Here's how the part is built. I have some questions about the finished solid (model axes, mm). Round coordinates to 2 decimals unless told otherwise and drop trailing zeros. Order: outer loops, then holes, each group sorted by start corner. A loop starts at its lowest first (then second) coordinate and runs counter-clockwise, first axis right, second up. Notation, with made-up numbers: M -19,-34.75 L 19,-34.75 A4 ccw 19,-27.75 Z; hole C 73.25,10.5 d1. An arc over 180 degrees is marked long. Answer as CSV lines item,"result". Start each with the question number.
```python
from build123d import *

# Parameters (mm, degrees)
SKETCH1_W          = 76.2
SKETCH1_H          = 44.45
BASE_FLANGE1_DEPTH = 4.55422
CUT_EXTRUDE1_DEPTH = 45.342998825
FILLET1_R          = 4.7625
FILLET2_R          = 12.7
SKETCH3_R          = 3.175
CUT_EXTRUDE2_DEPTH = 45.342998825
FILLET3_R          = 6.35
CUT_EXTRUDE3_DEPTH = 45.342998825


# Sheet-metal steps are written as plain solids
with BuildPart() as part:
    # Sketch1 → Base-Flange1 (new body)
    with BuildSketch(Plane.XY):
        Rectangle(SKETCH1_W, SKETCH1_H)
    extrude(amount=BASE_FLANGE1_DEPTH)

    # Sketch2 → Cut-Extrude1 (cut, through all)
    with BuildSketch(Plane.XY.offset(4.55422)):
        Polygon((12.7, 22.225), (38.1, 15.419090512), (38.1, 22.225), align=None)
    extrude(amount=-CUT_EXTRUDE1_DEPTH, mode=Mode.SUBTRACT)

    # Fillet1
    fillet1_edges = [part.edges().sort_by_distance(p)[0] for p in [
        (-38.1, 22.225, 2.27711),
    ]]
    fillet(fillet1_edges, radius=FILLET1_R)

    # Fillet2
    fillet2_edges = [part.edges().sort_by_distance(p)[0] for p in [
        (12.7, 22.225, 2.27711),
        (38.1, 15.419090512, 2.27711),
    ]]
    fillet(fillet2_edges, radius=FILLET2_R)

    # Sketch3 → Cut-Extrude2 (cut, through all)
    with BuildSketch(Plane.XY.offset(4.55422)):
        with Locations((0, -9.525)):
            Circle(SKETCH3_R)
        with Locations((25.4, -9.525)):
            Circle(SKETCH3_R)
    extrude(amount=-CUT_EXTRUDE2_DEPTH, mode=Mode.SUBTRACT)

    # Fillet3
    fillet3_edges = [part.edges().sort_by_distance(p)[0] for p in [
        (38.1, -22.225, 2.27711),
        (-38.1, -22.225, 2.27711),
    ]]
    fillet(fillet3_edges, radius=FILLET3_R)

    # Sketch4 → Cut-Extrude3 (cut, through all)
    with BuildSketch(Plane.XY.offset(4.55422)):
        with BuildLine():
            Line((-3.175, -9.525), (-3.175, -3.175))
            ThreePointArc((-3.175, -3.175), (0, 0), (3.175, -3.175))
            Line((3.175, -3.175), (3.175, -9.525))
            ThreePointArc((3.175, -9.525), (0, -12.7), (-3.175, -9.525))
        make_face()
        with BuildLine():
            Line((22.225, -9.525), (22.225, -3.175))
            ThreePointArc((22.225, -3.175), (25.4, 0), (28.575, -3.175))
            Line((28.575, -3.175), (28.575, -9.525))
            ThreePointArc((28.575, -9.525), (25.4, -12.7), (22.225, -9.525))
        make_face()
    extrude(amount=-CUT_EXTRUDE3_DEPTH, mode=Mode.SUBTRACT)


solid = part.part
```
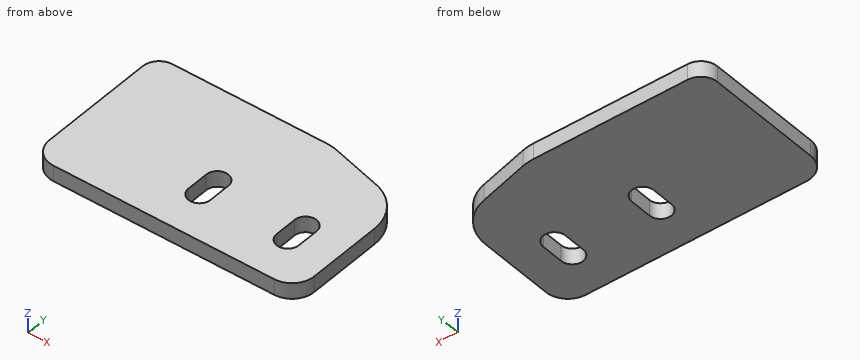
Item 1: If we section it at C-C on x = 25.4: Please give me the cut outline in (y, z) (3 decimals).
Item 2: If we section it at D-D on y = 11.5: Please give me the cut outline in (x, z), and give its area (3 significant figures).
Item 3: For P1, Ø1.5, axis at x = 22, z = 3, coming from the +Y side, with a flat end and sliding along its axis, tell me the tip position at first contact or that it passes through.
Item 4: If we section it at B-B on z = 1.45: Count the separate pieces of the cut face and the enclosed holes in it, and give its area (3 significant figures).
Item 5: If I drill on line 1 along X through (y, z) = (-12, 3.85); line 2 along X through (y, z) = (-11, 1.4); line 3 along Y through (x, z) = (24, 1.55) (3 decimals), over which ranges is the centre line in solid material (lowest first)?
Item 6: If we section it at A-A on x = 0: Please give me the cut outline in (y, z) (3 decimals).
Geometry says:
1,outline,"M -22.225,0 L -12.7,0 L -12.7,4.554 L -22.225,4.554 Z; M 0,0 L 18.822,0 L 18.822,4.554 L 0,4.554 Z"
2,outline,"M -38.1,0 L 36.68,0 L 36.68,4.55 L -38.1,4.55 Z"
2,area,"341 mm²"
3,P1,"y = 19.93"
4,separate pieces,"1"
4,enclosed holes,"2"
4,area,"3,120 mm²"
5,line 1,"-38.1 to -1.99, 1.99 to 23.41, 27.39 to 38.1"
5,line 2,"-38.1 to -2.81, 2.81 to 22.59, 28.21 to 38.1"
5,line 3,"-22.225 to -12.375, -0.325 to 19.197"
6,outline,"M -22.225,0 L -12.7,0 L -12.7,4.554 L -22.225,4.554 Z; M 0,0 L 22.225,0 L 22.225,4.554 L 0,4.554 Z"
